```python
from build123d import *

# Parameters (mm, degrees)
SKETCH1_W           = 77
SKETCH1_H           = 35
BOSS_EXTRUDE1_DEPTH = 7
SKETCH2_R           = 11.25
CUT_EXTRUDE1_DEPTH  = 15
SKETCH3_W           = 77
SKETCH3_H           = 15
BOSS_EXTRUDE2_DEPTH = 40
SKETCH4_R           = 2.1
CUT_EXTRUDE2_DEPTH  = 20
FILLET1_R           = 2
FILLET2_R           = 2


with BuildPart() as part:
    # Sketch1 → Boss-Extrude1 (new body)
    with BuildSketch(Plane.XY):
        with Locations((3.5, 0)):
            Rectangle(SKETCH1_W, SKETCH1_H)
    extrude(amount=BOSS_EXTRUDE1_DEPTH)

    # Sketch2 → Cut-Extrude1 (cut)
    with BuildSketch(Plane.XY.offset(7)):
        with Locations((0, -2.5)):
            Circle(SKETCH2_R)
    extrude(amount=-CUT_EXTRUDE1_DEPTH, mode=Mode.SUBTRACT)

    # Sketch3 → Boss-Extrude2 (add)
    with BuildSketch(Plane(origin=(0, 0, 0), x_dir=(-1, 0, 0), z_dir=(0, 0, -1))):
        with Locations((-3.5, -25)):
            Rectangle(SKETCH3_W, SKETCH3_H)
    extrude(amount=-BOSS_EXTRUDE2_DEPTH)

    # Sketch4 → Cut-Extrude2 (cut)
    with BuildSketch(Plane(origin=(0, -17.5, 0), x_dir=(1, 0, 0), z_dir=(0, 1, 0))):
        with Locations((-28, -35)):
            Circle(SKETCH4_R)
        with Locations((-28, -12)):
            Circle(SKETCH4_R)
        with Locations((35, -35)):
            Circle(SKETCH4_R)
        with Locations((35, -12)):
            Circle(SKETCH4_R)
    extrude(amount=-CUT_EXTRUDE2_DEPTH, mode=Mode.SUBTRACT)

    # Fillet1
    fillet1_edges = [part.edges().sort_by_distance(p)[0] for p in [
        (3.5, -17.5, 7),
    ]]
    fillet(fillet1_edges, radius=FILLET1_R)

    # Fillet2
    fillet2_edges = [part.edges().sort_by_distance(p)[0] for p in [
        (42, -25, 40),
        (-35, -25, 40),
        (3.5, -32.5, 0),
        (-35, 17.5, 3.5),
        (42, 17.5, 3.5),
    ]]
    fillet(fillet2_edges, radius=FILLET2_R)


solid = part.part
```
Design review of the part built by this model. Coordinates are the model's own, in mm. A direction names the side the tool comes from. Coordinates: 2 decimals unless noted, no trailing zeros. Write each loop counter-clockwise with the first axis right and the second up, starting at its lowest first coordinate (ties: lowest second). Pieces come first, ordered by that corner, then holes.
1) Add section C-C (z = 35). Write out the cut boundary in (x, y).
2) Add section A-A (x = 9). Write out the cut boundary in (y, z), plus the area to 4 significant figures.
3) To check wall thickness, follow L1, parallel to Z at x = 35, y = -26; L2, parallel to X at y = -20.75, z = 12; L3, parallel to Z at x = -24, y = -9.5. State the ranges of each line that lie inside material, in increasing order.
4) Mouldability with a two-part tool opening along Y and no side actions: class faces 1 (the cylindrical face through (33.334, -24.895, 36.278)), 2 (the cylindrical face through (-2.439, -13.482, 3.549)), 3 (the cylindrical face through (-34.4, 16.93, 3.55)) as +Y half, -Y half, draft (parallel to the pull), parting line (faces both ways), or undercut.
5) Machinability: for faces 4 (the flat face through (3, 9, 7)), 5 (the flat face through (-35, -20, 15)), which of the approach directions +Z, -Z, +X, -X, +Y, -Y give a long, thin tool a straight path to every point of the face, cutting with its end or side? Answer none if there is none.
6) Add section D-D (y = -12). Write out the cut boundary in (x, z), plus the area to 3 significant figures.
7) Insertion check: pin 1 (4 mm diameter, centred on x = 35, z = 35, fed in from +Y); pin 2 (6 mm diameter, centred on x = 13, y = -9, fed in from +Z); pin 3 (5 mm diameter, centred on x = -28, z = 12, fed in from +Y); pin 4 (1 mm diameter, centred on x = 19, y = -15.5, fed in from +Z). Each pin has a flat end and moves straight along its axis. Give the tip position at first contact, or say it passes through.
8) Add section B-B (y = -18.5). Write out the cut boundary in (x, z).
Check result:
1. outline: (-35, -32.5) - (-30.1, -32.5) - (-30.1, -17.5) - (-35, -17.5) - close; (-25.9, -32.5) - (32.9, -32.5) - (32.9, -17.5) - (-25.9, -17.5) - close; (37.1, -32.5) - (42, -32.5) - (42, -17.5) - (37.1, -17.5) - close
2. outline: (-32.5, 2) arc R2 ccw to (-30.5, 0) - (-9.25, 0) - (-9.25, 7) - (-15.5, 7) arc R2 cw to (-17.5, 9) - (-17.5, 40) - (-32.5, 40) - close; (4.25, 0) - (17.5, 0) - (17.5, 7) - (4.25, 7) - close
2. area: 750.5 mm2
3. L1: z = 0 to 9.9, 14.1 to 32.9, 37.1 to 40
3. L2: x = -35 to -30.1, -25.9 to 32.9, 37.1 to 42
3. L3: z = 0 to 7
4. face 1: draft
4. face 2: undercut
4. face 3: +Y half
5. face 4: +Z, +X, -X, +Y
5. face 5: +Z, -Z, -X, +Y, -Y
6. outline: (-35, 0) - (-6.03, 0) - (-6.03, 7) - (-35, 7) - close; (6.03, 0) - (42, 0) - (42, 7) - (6.03, 7) - close
6. area: 455 mm2
7. pin 1: passes through
7. pin 2: stops at z = 7
7. pin 3: stops at y = -17.5
7. pin 4: stops at z = 7.06
8. outline: (-35, 0) - (42, 0) - (42, 38) arc R2 ccw to (40, 40) - (-33, 40) arc R2 ccw to (-35, 38) - close; hole circle Ø4.2 at (-28, 12); hole circle Ø4.2 at (-28, 35); hole circle Ø4.2 at (35, 12); hole circle Ø4.2 at (35, 35)
